Autodesk Inventor part; units mm, degrees
ref_plane "Work Plane1" through (0, 0, 0) normal (0, 0, 1) x (1, 0, 0)
ref_plane "YZ Plane" through (0, 0, 0) normal (1, 0, 0) x (0, 1, 0)
ref_plane "XZ Plane" through (0, 0, 0) normal (0, 1, 0) x (-1, 0, 0)
ref_plane "Work Plane1" through (0, 0, 0) normal (0, 0, 1) x (1, 0, 0)
sketch "Sketch1" plane through (0, 0, 0) normal (0, 0, 1) x (1, 0, 0)
  line L0 (-13.9399, 12.3161) -> (-5.7696, 7.2832)
  line L1 (-15.6051, 9.6128) -> (-13.9399, 12.3161)
  line L2 (-7.4348, 4.5799) -> (-15.6051, 9.6128)
  line L3 (-5.7696, 7.2832) -> (-7.4348, 4.5799) construction
  line L4 (-5.4698, 3.3694) -> (-7.4348, 4.5799) construction
  line L5 (-3.8046, 6.0727) -> (1.6652, 2.7033)
  line L6 (-5.4698, 3.3694) -> (-3.8046, 6.0727) construction
  line L7 (0, 0) -> (-5.4698, 3.3694)
  line L8 (0, 0) -> (1.6652, 2.7033)
  line L9 (-5.3472, -249.9446) -> (-16.3579, -243.162)
  line L10 (-14.6927, -240.4587) -> (-3.682, -247.2413)
  line L11 (-16.3579, -243.162) -> (-14.6927, -240.4587) construction
  line L12 (-9.0019, -247.6933) -> (-20.2167, -240.7849) construction
  line L13 (-6.6483, -245.4141) -> (-18.5515, -238.0817) construction
  line L14 (0.5444, -249.8448) -> (0.5444, -249.8448)
  line L15 (0.5444, -2.2912) -> (0.5444, 0.8838) construction
  line L16 (0.5444, 0.8838) -> (0.5444, 0.8838) construction
  line L17 (0.5444, 0.8838) -> (0.5444, -253.0198) construction
  line L18 (0.5444, -253.0198) -> (0.5444, -253.0198) construction
  line L19 (0.5444, -253.0198) -> (0.5444, 0.8838) construction
  line L20 (0.5444, 0.8838) -> (0.5444, 0.8838) construction
  line L21 (0.5444, 0.8838) -> (0.5444, -2.2912) construction
  line L22 (0.5444, -2.2912) -> (0.5444, -2.2912) construction
  line L23 (-7.4904, 8.3432) -> (-9.1556, 5.6399)
  line L24 (-3.7491, 2.3094) -> (-2.0838, 5.0127)
  line L25 (0, 0) -> (0.5444, -0.3354)
  line L26 (0.5444, -0.3354) -> (0.5444, -253.0198)
  line L27 (-12.9719, -241.5187) -> (-14.6371, -244.222)
  line L28 (-15.6051, 9.6128) -> (-23.1742, 14.2754)
  line L29 (-23.1742, 14.2754) -> (-23.1742, -111.4572)
  line L30 (-25.9909, -237.228) -> (-24.3256, -234.5248) construction
  line L31 (-21.0892, -112.7416) -> (-23.1742, -111.4572) construction
  line L32 (-23.1742, -111.4572) -> (0.5444, -126.068) construction
  line L33 (-23.1742, -111.4572) -> (-24.8395, -114.1605) construction
  line L34 (-22.7544, -115.4449) -> (-24.8395, -114.1605) construction
  line L35 (-24.8395, -114.1605) -> (0.5444, -129.797) construction
  line L36 (-24.8395, -114.1605) -> (-24.8395, -234.2082)
  line L37 (-24.3256, -234.5248) -> (-24.8395, -234.2082) construction
  line L38 (-24.8395, -234.2082) -> (-18.5515, -238.0817)
  line L39 (-12.9719, -241.5187) -> (-4.6458, -228.0024)
  line L40 (-18.5515, -238.0817) -> (-10.2253, -224.5653)
  line L41 (-10.2253, -224.5653) -> (-4.6458, -228.0024)
  line L42 (-14.4373, -243.8976) -> (-5.1474, -249.6202)
  line L43 (1.4654, 2.3789) -> (-2.2837, 4.6883)
  line L44 (-7.6902, 8.0188) -> (-14.1397, 11.9917)
  line L45 (0.5444, -122.6898) -> (3.3735, -122.6898) construction
  line L46 (0.5444, -129.4462) -> (3.3735, -129.4462) construction
  line L47 (-3.7491, 2.3094) -> (-12.0752, -11.2069)
  line L48 (-12.0752, -11.2069) -> (-17.4817, -7.8765)
  line L49 (-17.4817, -7.8765) -> (-9.1556, 5.6399)
  line L50 (-14.7785, -9.5417) -> (-4.7871, 6.6779) construction
  line L51 (-15.8457, -0.6803) -> (-6.3842, -6.5086)
  line L52 (-6.3842, -6.5086) -> (-3.7199, -2.1834)
  line L53 (-3.7199, -2.1834) -> (-13.1813, 3.6449)
  line L54 (-13.1813, 3.6449) -> (-15.8457, -0.6803)
  line L55 (-15.8457, -0.6803) -> (-3.7199, -2.1834) construction
  line L56 (-6.3842, -6.5086) -> (-13.1813, 3.6449) construction
  line L57 (-7.4356, -226.2838) -> (-17.4269, -242.5035) construction
  line L58 (-18.4941, -233.6421) -> (-9.0327, -239.4704)
  line L59 (-9.0327, -239.4704) -> (-6.3683, -235.1452)
  line L60 (-6.3683, -235.1452) -> (-15.8298, -229.3169)
  line L61 (-15.8298, -229.3169) -> (-18.4941, -233.6421)
  line L62 (-18.4941, -233.6421) -> (-6.3683, -235.1452) construction
  line L63 (-9.0327, -239.4704) -> (-15.8298, -229.3169) construction
  line L64 (0.5444, -122.6898) -> (-15.6765, -122.6898)
  line L65 (-15.6765, -122.6898) -> (-15.6765, -129.4462)
  line L66 (-15.6765, -129.4462) -> (0.5444, -129.4462)
  line L67 (3.3735, -126.068) -> (-15.6765, -126.068) construction
  line L68 (-8.6915, -131.6242) -> (-8.6915, -120.5117)
  line L69 (-8.6915, -120.5117) -> (-3.6115, -120.5117)
  line L70 (-3.6115, -120.5117) -> (-3.6115, -131.6242)
  line L71 (-3.6115, -131.6242) -> (-8.6915, -131.6242)
  line L72 (-8.6915, -131.6242) -> (-3.6115, -120.5117) construction
  line L73 (-8.6915, -120.5117) -> (-3.6115, -131.6242) construction
  line L74 (-24.8395, -114.1605) -> (-10.9932, -122.6898)
  line L75 (-23.1742, -111.4572) -> (-8.4754, -120.5117)
  line L76 (-16.6864, -115.4537) -> (-18.3516, -118.157)
  line L77 (-20.1943, 16.1688) -> (-21.8595, 13.4656) construction
  line L78 (-21.8595, 13.4656) -> (-23.1742, 11.3313)
  line L79 (-23.2443, -111.414) -> (-24.9095, -114.1173)
  line L80 (-3.6115, -131.6242) -> (0.5444, -131.6242)
  line L81 (-3.6115, -120.5117) -> (0.5444, -120.5117)
  line L82 (-3.682, -247.2413) -> (0.5444, -249.8448)
  line L83 (-5.3472, -249.9446) -> (-3.682, -247.2413)
  line L84 (-22.6481, -239.2872) -> (-20.9829, -236.5839)
  line L85 (-18.3229, -241.9515) -> (-22.6481, -239.2872)
  line L86 (-18.5515, -238.0817) -> (-20.2167, -240.7849)
  line L87 (-20.0168, -240.4606) -> (-22.4483, -238.9628)
  line L88 (0.5444, -122.6898) -> (0.5444, -129.4462)
  line L89 (0.5444, -122.6898) -> (0.5444, -129.4462)
  line L90 (3.3735, -122.6898) -> (3.3735, -129.4462)
  line L91 (-3.8046, 6.0727) -> (-5.7696, 7.2832)
  point P0 (-6.4523, 3.9747)
  point P1 (-9.7828, -1.4319)
  point P2 (-12.4312, -234.3936)
  point P3 (-6.1515, -126.068)
  point P4 (-16.5532, -234.8378)
  point P5 (-13.8888, -230.5125)
  point P6 (-8.3093, -233.9495)
  point P7 (-10.9736, -238.2748)
  point P8 (0.5444, -129.4462)
  point P9 (-3.6115, -129.4462)
  point P10 (-8.6915, -129.4462)
  point P11 (-8.6915, -122.6898)
  point P12 (-3.6115, -122.6898)
  point P13 (0.5444, -122.6898)
  point P14 (-5.7473, -0.9345)
  point P15 (-8.4117, -5.2597)
  point P16 (-13.8182, -1.9293)
  point P17 (-11.1539, 2.396)
  dimension "d0" = 3.175
  dimension "d1" = 3.175
  dimension "d2" = 2.021
  dimension "d3" = 2.021
  dimension "d5" = 19.05
  dimension "d7" = 0.381
  dimension "d8" = 0.381
  dimension "d10" = 8.89
  dimension "d11" = 11.1125
  dimension "d12" = 5.08
  dimension "d13" = 11.1125
  dimension "d14" = 5.08
  dimension "d15" = 19.05
  dimension "d16" = 11.1125
  dimension "d17" = 5.08
  dimension "d18" = 7.62
  dimension "d21" = 0.381
  dimension "d22" = 19.05
extrude "Extrusion1" add sketch "Sketch1" along normal blind 6.35 contours L44 L23 L2 L1 | L2 L49 L53 L54 L51 L48 L47 L52 L7 L25 L26 L81 L69 L75 L29 L78 L28 | L43 L8 L7 L24 | L75 L69 L68 L64 L74 L76 | L74 L64 L65 L66 L68 L71 L80 L26 L82 L10 L39 L58 L59 L60 L41 L40 L61 L38 L36 | L81 L26 L64 L70 | L66 L26 L80 L70 | L38 L86 L87 L84 | L83 L42 L27 L10
equation "\"d3\" = d2"
properties part number "Inner Bracket" material "Polycarbonate, Clear"
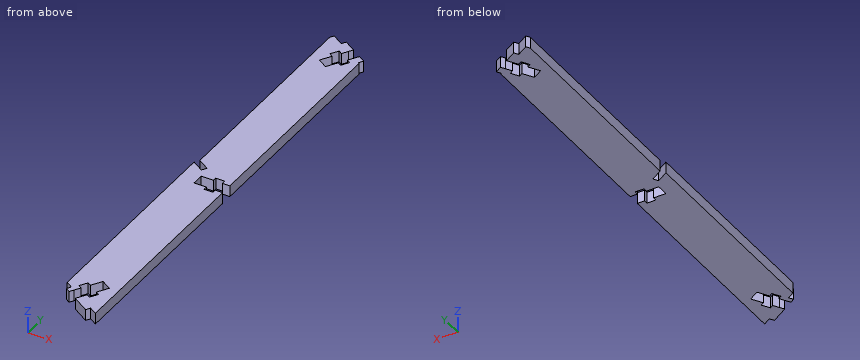
Verification items for the finished model (mm, model axes). Coordinates: 2 decimals unless noted, no trailing zeros. Loops run counter-clockwise (first coordinate to the right, second up) from the corner with the lowest first, then second, coordinate; pieces in that order, holes last. Notation, with made-up numbers: (39, 14.25) - (94, 14.25) arc R21 cw to (94, 53.25) - close; hole circle Ø7 at (58.5, 42). An arc over 180 degrees is marked (long way). Put each result on its own line as item: value.
Item 1: Gauge pin test, flat ends, axial feed: pin 1 Ø3 at (x, z) = (-14, 2) entering from +Y; pin 2 Ø3 at (y, z) = (-211.5, 2) entering from +X; pin 3 Ø3 at (y, z) = (-40.5, 2) entering from -X. Record the tip position at first contact, or that the pin passes through.
Conclusion:
pin 1: stops at y = 11.99
pin 2: stops at x = 0.54
pin 3: stops at x = -23.17
Item 2: Scan lines: line 1 along Y through (x, z) = (-22.25, 4.75); line 2 along Y through (x, z) = (-11.5, 5); line 3 along Y through (x, z) = (-12.75, 1.75). Record each from-to range of solid material in increasing order.
Conclusion:
line 1: y = -239.08 to -238.64, -235.8 to -115.76, -112.03 to 12.83
line 2: y = -245.71 to -239.13, -226.63 to -129.45, -122.69 to -10.27, 2.61 to 10.37
line 3: y = -244.94 to -241.16, -228.66 to -129.45, -122.69 to -10.79, 3.38 to 11.14
Item 3: Section check A-A (y = -53). Enter the section's corners in (x, z).
Conclusion:
outline: (-23.17, 0) - (0.54, 0) - (0.54, 6.35) - (-23.17, 6.35) - close
Item 4: Section check B-B (y = -165). Enter the section's corners in (x, z), then the cut area to 3 significant figures.
Conclusion:
outline: (-24.84, 0) - (0.54, 0) - (0.54, 6.35) - (-24.84, 6.35) - close
area: 161 mm2
